Geometry check sheet. Reference: the model listing, model coordinates, mm. Face numbers are marked on the shaded views. A direction names the side the tool comes from. Round coordinates to 2 decimals unless told otherwise and drop trailing zeros. Order: outer loops, then holes, each group sorted by start corner. A loop starts at its lowest first (then second) coordinate and runs counter-clockwise, first axis right, second up. Notation, with made-up numbers: (69.25, -16.75) - (97.25, -16.75) arc R22 cw to (97.25, 1.25) - close; hole circle Ø10 at (71.25, -14). An arc over 180 degrees is marked (long way). Return JSON: item names as keys, results as strings. Group by question number.
Q1. Sectioned sample at B-B, the plane x = 11. Record the cut outline in (y, z), then the cut area to 3 significant figures.
Q2. Tool access check on the marked faces 4, 5, 6, 7 and 8. Record the directions out of +Z, -Z, +X, -X, +Y, -Y that give a thin tool (end or side, any length) a straight path to the whole face; none if there is none.
Q3. Sectioned sample at D-D, the plane y = 6.5. Record the cut outline in (x, z).
Q4. Sectioned sample at C-C, the plane z = 7.5. Give the number of separate pieces and of enclosed holes in the cut face, then the cut area to 3 significant figures.
Q5. Sectioned sample at A-A, the plane y = 1.5. Record the cut outline in (x, z), then the cut area to 3 significant figures.
Q6. Material ranges on line 1 along Z through (x, y) = (-11, 0.55); line 2 along X through (y, z) = (2, 10); line 3 along Y through (x, z) = (-13, 12.25), recorded low to high.
Q7. Gauge pin test, flat ends, axial feed: pin 1 Ø2 at (y, z) = (4.5, 7.5) entering from -X; pin 2 Ø2 at (x, z) = (-0.5, 11) entering from -Y; pin 3 Ø2 at (y, z) = (10, 8) entering from +X. Record the tip position at first contact, or that the pin passes through.
Q8. Draft check along X on the marked faces 1, 2 and 3. Enter one of: pulls with the +X half, pulls with the -X half, needs draft (parallel to the pull), parting line crosses it, or undercut.
```python
from build123d import *

# Parameters (mm, degrees)
F1_DEPTH       = 15
F4_D           = 3
F4_DEPTH       = 3
F4_CSINK_D     = 5
F4_CSINK_ANGLE = 90
F4_TIP         = 0.9012909285


with BuildPart() as f1:
    # F0 (on Top) → F1 (new body)
    with BuildSketch(Plane.XY):
        with BuildLine():
            Line((5, 7), (5, 0))
            Line((5, 0), (15, 0))
            Line((15, 0), (15, 2))
            ThreePointArc((15, 2), (14.7071067812, 2.7071067812), (14, 3))
            Line((14, 3), (8, 3))
            Line((8, 3), (8, 10))
            ThreePointArc((8, 10), (7.1213203436, 12.1213203436), (5, 13))
            Line((5, 13), (0, 13))
            Line((0, 13), (0, 10))
            Line((0, 10), (2, 10))
            ThreePointArc((2, 10), (4.1213203436, 9.1213203436), (5, 7))
        make_face()
        with BuildLine():
            Line((-2, 10), (0, 10))
            Line((0, 10), (0, 13))
            Line((0, 13), (-5, 13))
            ThreePointArc((-5, 13), (-7.1213203436, 12.1213203436), (-8, 10))
            Line((-8, 10), (-8, 3))
            Line((-8, 3), (-14, 3))
            ThreePointArc((-14, 3), (-14.7071067812, 2.7071067812), (-15, 2))
            Line((-15, 2), (-15, 0))
            Line((-15, 0), (-5, 0))
            Line((-5, 0), (-5, 7))
            ThreePointArc((-5, 7), (-4.1213203436, 9.1213203436), (-2, 10))
        make_face()
    extrude(amount=F1_DEPTH)

    # F4
    with Locations(Plane(origin=(0, 3, 0), x_dir=(1, 0, 0), z_dir=(0, 1, 0))):
        with Locations((11, -7.5), (-11, -7.5)):
            CounterSinkHole(F4_D / 2, F4_CSINK_D / 2, depth=F4_DEPTH, counter_sink_angle=F4_CSINK_ANGLE)
            with Locations((0, 0, -(F4_DEPTH + F4_TIP / 2))):  # 118° drill point
                Cone(0, F4_D / 2, F4_TIP, mode=Mode.SUBTRACT)


solid = f1.part
```
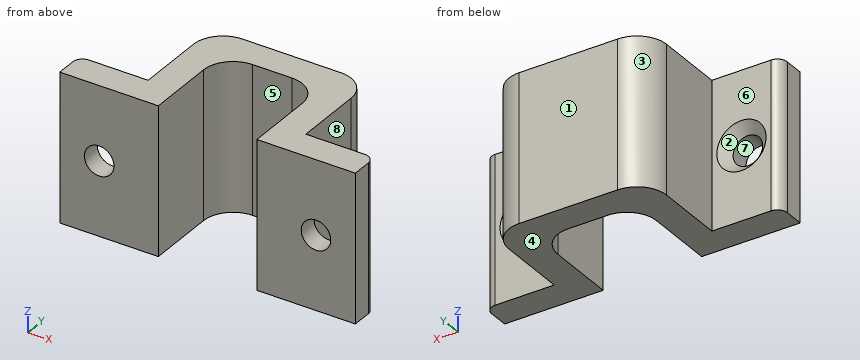
Reply:
{
 "1": {"outline": "(0, 0) - (3, 0) - (3, 5) - (2, 6) - (0, 6) - close; (0, 9) - (2, 9) - (3, 10) - (3, 15) - (0, 15) - close", "area": "35.0 mm^2"},
 "2": {"face 4": "-Z, +X, -X, +Y, -Y", "face 5": "+Z, -Z, -Y", "face 6": "+Z, -Z, -X, +Y", "face 7": "+Y, -Y", "face 8": "+Z, -Z, +X, +Y"},
 "3": {"outline": "(-8, 0) - (-5, 0) - (-5, 15) - (-8, 15) - close; (5, 0) - (8, 0) - (8, 15) - (5, 15) - close"},
 "4": {"separate pieces": "3", "enclosed holes": "0", "area": "130 mm^2"},
 "5": {"outline": "(-15, 0) - (-5, 0) - (-5, 15) - (-15, 15) - close; (5, 0) - (15, 0) - (15, 15) - (5, 15) - close; hole circle Ø3 at (-11, 7.5); hole circle Ø3 at (11, 7.5)", "area": "286 mm^2"},
 "6": {"line 1": "0 to 6, 9 to 15", "line 2": "-15 to -5, 5 to 15", "line 3": "0 to 3"},
 "7": {"pin 1": "x = -8", "pin 2": "y = 10", "pin 3": "x = 8"},
 "8": {"face 1": "needs draft", "face 2": "undercut", "face 3": "pulls with the -X half"}
}
